Could you check a few things on this model? Use its own coordinates, in mm. Face numbers are marked on the shaded views. Coordinates: 2 decimals unless noted, no trailing zeros. Order: outer loops, then holes, each group sorted by start corner. A loop starts at its lowest first (then second) coordinate and runs counter-clockwise, first axis right, second up.
```python
from build123d import *


with BuildPart() as part:
    # Esquisse2 → Révolution1 (revolve)
    with BuildSketch(Plane.XY, mode=Mode.PRIVATE) as r_volution1_sk:
        with BuildLine():
            Line((380, 150), (380, 80))
            Line((380, 80), (0, 80))
            Line((0, 80), (0, 150))
            Line((0, 150), (30, 150))
            Line((30, 150), (30, 145))
            ThreePointArc((30, 145), (38.786796564, 123.786796564), (60, 115))
            Line((60, 115), (80, 115))
            Line((80, 115), (80, 105))
            Line((80, 105), (110, 105))
            Line((110, 105), (110, 115))
            Line((110, 115), (270, 115))
            Line((270, 115), (270, 105))
            Line((270, 105), (300, 105))
            Line((300, 105), (300, 115))
            Line((300, 115), (320, 115))
            ThreePointArc((320, 115), (341.213203436, 123.786796564), (350, 145))
            Line((350, 145), (350, 150))
            Line((350, 150), (380, 150))
        make_face()
    revolve(r_volution1_sk.sketch.rotate(Axis((0, 0, 0), (1, 0, 0)), 90), axis=Axis((0, 0, 0), (1, 0, 0)))


solid = part.part
```
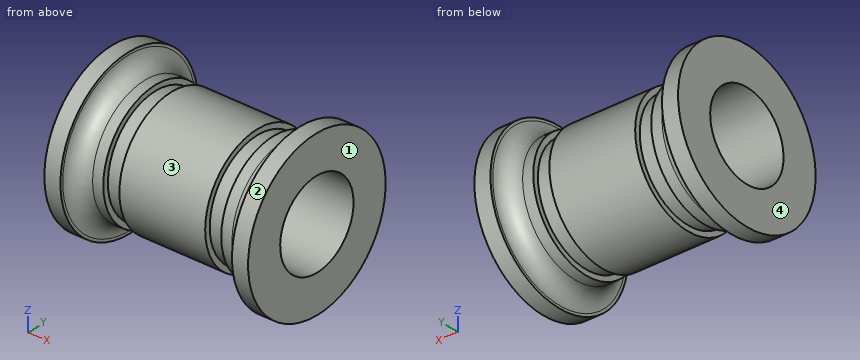
Item 1: Suppose I cut it at A-A (x = 200.5). List the corners of the cut face in (y, z) for me, and give its area (3 significant figures).
Item 2: For pin 1 Ø12 at (x, y) = (307, 2) entering from +Z; pin 2 Ø8 at (x, y) = (301.5, 71) entering from +Z; pin 3 Ø4 at (x, y) = (116.5, 8) entering from +Z, each with a flat end and sliding along its axis, tell me the tip position at first contact or that it passes through.
Item 3: I need wall thicknesses on line 1 (X direction, y = -100, z = -51); line 2 (Y direction, x = 171, z = 0); line 3 (Y direction, x = 100, z = 0). Which ranges of each line are inside material? Lowest first, please.
Item 4: Thinking about a two-plate mould opening in X: for the marked faces 1, 2, 3 and 4, which applies, +X half, -X half, draft (parallel to the pull), parting line (faces both ways), or undercut?
Geometry results:
1. outline: circle Ø230 at (0, 0); hole circle Ø160 at (0, 0)
1. area: 21,400 mm2
2. pin 1: stops at z = 115
2. pin 2: stops at z = 93.47
2. pin 3: stops at z = 114.84
3. line 1: x = 0 to 80, 110 to 270, 300 to 380
3. line 2: y = -115 to -80, 80 to 115
3. line 3: y = -105 to -80, 80 to 105
4. face 1: +X half
4. face 2: draft
4. face 3: undercut
4. face 4: -X half
